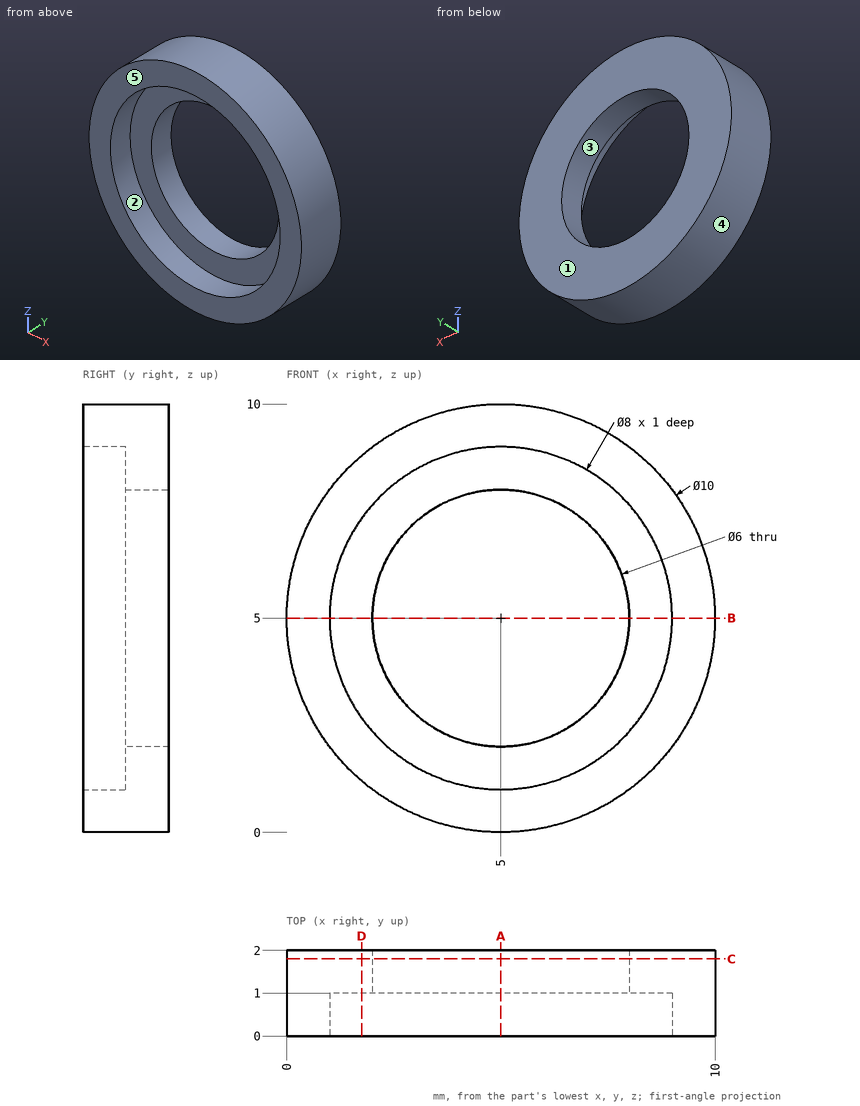
Study the drawing (mm; zero at the part's minimum x, y, z) and answer. A direction names the side the tool comes from. Give positions to 0.01 mm unless a question says otherwise; leave off trailing zeros. Order: outer loops, then holes, each group sorted by start corner. A loop starts at its lowest first (then second) coordinate and runs counter-clockwise, first axis right, second up.
1) Find section A-A on x = 5. Write down the section's boundary in (y, z).
Reported:
outline: (0, 0) - (2, 0) - (2, 2) - (1, 2) - (1, 1) - (0, 1) - close; (0, 9) - (1, 9) - (1, 8) - (2, 8) - (2, 10) - (0, 10) - close
2) Find section B-B on z = 5. Write down the section's boundary in (x, y), then the cut area to 3 significant figures.
Reported:
outline: (0, 0) - (1, 0) - (1, 1) - (2, 1) - (2, 2) - (0, 2) - close; (8, 1) - (9, 1) - (9, 0) - (10, 0) - (10, 2) - (8, 2) - close
area: 6.00 mm2
3) Consider line 1 along X through (y, z) = (1.7, 5); line 2 along Y through (x, z) = (3, 2.5); line 3 along X through (y, z) = (1.45, 4.25). Determine where each line is inside the solid, lowest interval first.
Reported:
line 1: x = 0 to 2, 8 to 10
line 2: y = 1 to 2
line 3: x = 0.06 to 2.1, 7.9 to 9.94
4) Find section D-D on x = 1.75. Write down the section's boundary in (y, z), then the cut area to 3 significant figures.
Reported:
outline: (0, 1.2) - (2, 1.2) - (2, 8.8) - (0, 8.8) - (0, 7.33) - (1, 7.33) - (1, 2.67) - (0, 2.67) - close
area: 10.5 mm2
5) Find section C-C on y = 1.8. Write down the section's boundary in (x, z), then the cut area to 3 significant figures.
Reported:
outline: circle Ø10 at (5, 5); hole circle Ø6 at (5, 5)
area: 50.3 mm2
6) Determine the mould class of the marked faces 3, 4 and 5 for opening direction X: pulls with the +X half, pulls with the -X half, needs draft (parallel to the pull), parting line crosses it, or undercut.
Reported:
face 3: undercut
face 4: parting line crosses it
face 5: needs draft
7) For the marked faces 1 and 2, determine the directions among +Z, -Z, +X, -X, +Y, -Y from which every point of the face is accessible in a straight line to the end or side of a thin tool.
Reported:
face 1: +Z, -Z, +X, -X, +Y
face 2: -Y
